Can you work these out from the model? Positions are in its coordinate system, mm. A direction names the side the tool comes from. Coordinates: 2 decimals unless noted, no trailing zeros. Loops run counter-clockwise (first coordinate to the right, second up) from the corner with the lowest first, then second, coordinate; pieces in that order, holes last.
```python
from build123d import *

# Parameters (mm, degrees)
BOSS_EXTRUDE1_DEPTH   = 17.78
BOSS_EXTRUDE1_2_DEPTH = 17.78
BOSS_EXTRUDE1_3_DEPTH = 17.78
BOSS_EXTRUDE1_4_DEPTH = 17.78
BOSS_EXTRUDE1_5_DEPTH = 17.78
BOSS_EXTRUDE1_6_DEPTH = 17.78
BOSS_EXTRUDE2_DEPTH   = 7.62


with BuildPart() as part:
    # Sketch1 → Boss-Extrude1 (new body)
    with BuildSketch(Plane.XY):
        with BuildLine():
            Line((-63.5, 0.762), (-38.022245391, 0.762))
            ThreePointArc((-38.022245391, 0.762), (-31.409051973, 4.854056156), (-32.119852619, 12.598345226))
            Line((-32.119852619, 12.598345226), (-38.427776706, 20.532214336))
            Line((-38.427776706, 20.532214336), (-27.33774172, 20.532214336))
            Line((-27.33774172, 20.532214336), (-27.33774172, 0.762))
            Line((-27.33774172, 0.762), (-17.932333685, 0.762))
            Line((-17.932333685, 0.762), (-17.932333685, 20.532214336))
            Line((-17.932333685, 20.532214336), (-7.881253338, 20.532214336))
            Line((-7.881253338, 20.532214336), (-7.881253338, 29.930214336))
            Line((-7.881253338, 29.930214336), (-42.276317647, 29.930214336))
            ThreePointArc((-42.276317647, 29.930214336), (-48.598760185, 24.736726392), (-47.348213221, 16.650829474))
            Line((-47.348213221, 16.650829474), (-42.18759625, 10.16))
            Line((-42.18759625, 10.16), (-63.5, 10.16))
            Line((-63.5, 10.16), (-63.5, 0.762))
        make_face()
    extrude(amount=BOSS_EXTRUDE1_DEPTH)



with BuildPart() as body_2:
    # Sketch1 → Boss-Extrude1 2 (new body)
    with BuildSketch(Plane.XY):
        Polygon((11.051079885, 6.067535635), (13.004416536, 0.762), (23.01912578, 0.762), (12.280277522, 29.930214336), (-2.050542709, 29.930214336), (-13.385046463, 0.762), (-3.302420584, 0.762), (-1.240737517, 6.067535635), align=None)
        Polygon((5.071020227, 22.310214336), (0.733304445, 11.147535635), (9.180778587, 11.147535635), align=None, mode=Mode.SUBTRACT)
    extrude(amount=BOSS_EXTRUDE1_2_DEPTH)


with BuildPart() as body_3:
    # Sketch1 → Boss-Extrude1 3 (new body)
    with BuildSketch(Plane.XY):
        with BuildLine():
            ThreePointArc((43.443733283, 11.869404165), (43.556066702, 11.637854646), (43.712774585, 11.43370613))
            Line((43.712774585, 11.43370613), (44.162226788, 10.95718914))
            ThreePointArc((44.162226788, 10.95718914), (45.003789062, 10.367797223), (46.009984972, 10.16))
            Line((46.009984972, 10.16), (73.255000443, 10.16))
            Line((73.255000443, 10.16), (73.255000443, 0.762))
            Line((73.255000443, 0.762), (46.72115082, 0.762))
            ThreePointArc((46.72115082, 0.762), (45.463753928, 0.920074253), (44.28460982, 1.384459427))
            Line((44.28460982, 1.384459427), (43.705112819, 1.7012189))
            ThreePointArc((43.705112819, 1.7012189), (40.598056426, 3.858045423), (38.01751427, 6.623276383))
            Line((38.01751427, 6.623276383), (33.528766448, 12.598345226))
            Line((33.528766448, 12.598345226), (33.528766448, 0.762))
            Line((33.528766448, 0.762), (23.991875044, 0.762))
            Line((23.991875044, 0.762), (23.991875044, 29.930214336))
            Line((23.991875044, 29.930214336), (33.521137043, 29.930214336))
            Line((33.521137043, 29.930214336), (43.884526544, 29.930214336))
            ThreePointArc((43.884526544, 29.930214336), (52.294019037, 20.754281762), (43.366111034, 12.081925607))
            Line((43.366111034, 12.081925607), (43.443733283, 11.869404165))
        make_face()
        with BuildLine():
            ThreePointArc((41.080111034, 18.914029667), (43.179680202, 21.013598834), (41.080111034, 23.113168002))
            Line((41.080111034, 23.113168002), (33.525986314, 23.113168314))
            Line((33.525986314, 23.113168314), (33.525986314, 18.914029667))
            Line((33.525986314, 18.914029667), (41.080111034, 18.914029667))
        make_face(mode=Mode.SUBTRACT)
    extrude(amount=BOSS_EXTRUDE1_3_DEPTH)


with BuildPart() as body_4:
    # Sketch1 → Boss-Extrude1 4 (new body)
    with BuildSketch(Plane.XY):
        with BuildLine():
            ThreePointArc((30.671195496, -18.911591325), (30.783528915, -19.143140844), (30.940236798, -19.347289359))
            Line((30.940236798, -19.347289359), (31.389689001, -19.82380635))
            ThreePointArc((31.389689001, -19.82380635), (32.231251275, -20.413198267), (33.237447184, -20.62099549))
            Line((33.237447184, -20.62099549), (54.549850935, -20.62099549))
            Line((54.549850935, -20.62099549), (49.389233963, -14.130166015))
            ThreePointArc((49.389233963, -14.130166015), (48.27077915, -5.719302433), (55.156904328, -0.762))
            Line((55.156904328, -0.762), (73.255000443, -0.762))
            Line((73.255000443, -0.762), (73.255000443, -10.248781153))
            Line((73.255000443, -10.248781153), (59.020836327, -10.248781153))
            Line((59.020836327, -10.248781153), (65.328760414, -18.182650263))
            ThreePointArc((65.328760414, -18.182650263), (66.03956106, -25.926939334), (59.426367642, -30.01899549))
            Line((59.426367642, -30.01899549), (33.948613033, -30.01899549))
            ThreePointArc((33.948613033, -30.01899549), (32.69121614, -29.860921236), (31.512072033, -29.396536062))
            Line((31.512072033, -29.396536062), (30.932575032, -29.079776589))
            ThreePointArc((30.932575032, -29.079776589), (27.825518639, -26.922950067), (25.244976483, -24.157719107))
            Line((25.244976483, -24.157719107), (20.756228661, -18.182650263))
            Line((20.756228661, -18.182650263), (20.756228661, -30.01899549))
            Line((20.756228661, -30.01899549), (11.219337256, -30.01899549))
            Line((11.219337256, -30.01899549), (11.219337256, -0.762))
            Line((11.219337256, -0.762), (31.111988756, -0.762))
            ThreePointArc((31.111988756, -0.762), (39.610601796, -10.010542083), (30.625924739, -18.787644819))
            Line((30.625924739, -18.787644819), (30.671195496, -18.911591325))
        make_face()
        with BuildLine():
            ThreePointArc((28.307573247, -12.053626898), (30.407142414, -9.954057774), (28.307573334, -7.854488563))
            Line((28.307573334, -7.854488563), (20.753448527, -7.85448825))
            Line((20.753448527, -7.85448825), (20.753448527, -12.053626898))
            Line((20.753448527, -12.053626898), (28.307573247, -12.053626898))
        make_face(mode=Mode.SUBTRACT)
    extrude(amount=BOSS_EXTRUDE1_4_DEPTH)


with BuildPart() as body_5:
    # Sketch1 → Boss-Extrude1 5 (new body)
    with BuildSketch(Plane.XY):
        Polygon((-1.719438494, -24.713459854), (0.233898158, -30.01899549), (10.246907832, -30.01899549), (-0.524626942, -0.762), (-14.788261104, -0.762), (-26.15726441, -30.01899549), (-16.072938963, -30.01899549), (-14.011255896, -24.713459854), align=None)
        Polygon((-7.701197721, -8.655916551), (-12.038913502, -19.818595252), (-3.591439361, -19.818595252), align=None, mode=Mode.SUBTRACT)
    extrude(amount=BOSS_EXTRUDE1_5_DEPTH)


with BuildPart() as body_6:
    # Sketch1 → Boss-Extrude1 6 (new body)
    with BuildSketch(Plane.XY):
        Polygon((-50.396276017, -10.825946893), (-53.629040398, -0.762), (-63.5, -0.762), (-54.102, -30.01899549), (-44.704, -30.01899549), (-41.933974753, -21.395605814), (-39.163949505, -30.01899549), (-29.765949505, -30.01899549), (-20.367949505, -0.762), (-30.238909107, -0.762), (-34.002210372, -12.477565879), (-37.765511637, -0.762), (-47.163511637, -0.762), align=None)
    extrude(amount=BOSS_EXTRUDE1_6_DEPTH)


with BuildPart() as part_1:
    add(part.part)

    add(body_2.part)  # Boss-Extrude2 merges body 2

    add(body_3.part)  # Boss-Extrude2 merges body 3

    add(body_4.part)  # Boss-Extrude2 merges body 4

    add(body_5.part)  # Boss-Extrude2 merges body 5

    add(body_6.part)  # Boss-Extrude2 merges body 6
    # Sketch2 → Boss-Extrude2 (add)
    with BuildSketch(Plane.XY):
        with BuildLine():
            Line((-55.151201275, -31.516967273), (-65.434483981, -0.083873468))
            Line((-65.434483981, -0.083873468), (-65.434483981, 12.305447779))
            Line((-65.434483981, 12.305447779), (-47.078741234, 12.305447779))
            Line((-47.078741234, 12.305447779), (-49.980640842, 15.906912471))
            ThreePointArc((-49.980640842, 15.906912471), (-51.234201523, 26.666707013), (-42.069273563, 32.441539344))
            Line((-42.069273563, 32.441539344), (46.103426171, 32.441539344))
            ThreePointArc((46.103426171, 32.441539344), (54.623601335, 23.874155401), (51.136703514, 12.305447779))
            Line((51.136703514, 12.305447779), (75.860238392, 12.305447779))
            Line((75.860238392, 12.305447779), (75.860238392, -11.870528257))
            Line((75.860238392, -11.870528257), (62.378876642, -11.870528257))
            Line((62.378876642, -11.870528257), (67.089261913, -17.64019673))
            ThreePointArc((67.089261913, -17.64019673), (68.184246101, -26.660573767), (60.504295946, -31.516967273))
            Line((60.504295946, -31.516967273), (-55.151201275, -31.516967273))
        make_face()
    extrude(amount=BOSS_EXTRUDE2_DEPTH)


solid = part_1.part
```
(1) If we mould it in two halves opening along X, with no side actions, what happens to faces 1 (the flat face through (-48.757, -5.724, 12.629)), 2 (the cylindrical face through (-48.555, 24.848, 12.629)), 3 (the flat face through (73.255, -5, 13)), 4 (the flat face through (5, 6.068, 13))? For each: released by +X, released by -X, zero draft, split by the parting line, or undercut.
Check values:
face 1: undercut
face 2: released by -X
face 3: released by +X
face 4: undercut
(2) I want a section at C-C on x = 6.5. Write out the boundary of the cut face in (y, z), then the cut area to 3 significant figures.
Check values:
outline: (-31.52, 0) - (32.44, 0) - (32.44, 7.62) - (29.93, 7.62) - (29.93, 17.78) - (18.43, 17.78) - (18.43, 7.62) - (11.15, 7.62) - (11.15, 17.78) - (6.07, 17.78) - (6.07, 7.62) - (-19.84, 7.62) - (-19.84, 17.78) - (-30.02, 17.78) - (-30.02, 7.62) - (-31.52, 7.62) - close
area: 759 mm2
(3) I want a section at B-B on z = 15.75. State how many separate pieces and enclosed holes the cut face has, then the cut area to 3 significant figures.
Check values:
separate pieces: 6
enclosed holes: 4
area: 5,260 mm2
(4) If I drill on probe 1 along X at (y, z) = (-24, 9.25); probe 2 along Y at (x, z) = (61, 15.75); probe 3 along X at (y, z) = (17, 15.5), over which ranges is the centre line in solid material (lowest first)?
Check values:
probe 1: x = -56.04 to -42.77, -41.1 to -27.83, -23.82 to 8.03, 11.22 to 20.76, 25.13 to 66.69
probe 2: y = -29.85 to -12.74, -10.25 to -0.76, 0.76 to 10.16
probe 3: x = -47.61 to -35.62, -27.34 to -17.93, -7.08 to 3.01, 7.03 to 17.04, 23.99 to 51.35
(5) I'm going to push flat-ended pins straight in: pin 1 (12 mm diameter, centred on x = -51, y = 9.5, fed in from -Z); pin 2 (5 mm diameter, centred on y = 15, z = 15, fed in from -X); pin 3 (10 mm diameter, centred on y = 26, z = 4, fed in from +X); pin 4 (8 mm diameter, centred on y = 22, z = 11.5, fed in from -X). Where does each tip first touch, or does it pass through?
Check values:
pin 1: stops at z = 0
pin 2: stops at x = -47.94
pin 3: stops at x = 54.98
pin 4: stops at x = -52.23
(6) I want a section at A-A on z = 2. Write out the boundary of the cut face in (x, y), then the cut area to 3 significant figures.
Check values:
outline: (-65.43, -0.08) - (-55.15, -31.52) - (60.5, -31.52) arc R8.5 ccw to (67.09, -17.64) - (62.38, -11.87) - (75.86, -11.87) - (75.86, 12.31) - (51.14, 12.31) arc R11.8 ccw to (46.1, 32.44) - (-42.07, 32.44) arc R10.16 ccw to (-49.98, 15.91) - (-47.08, 12.31) - (-65.43, 12.31) - close
area: 7,930 mm2
(7) I want a section at D-D on y = 14. Write out the boundary of the cut face in (x, z), then the cut area to 3 significant figures.
Check values:
outline: (-48.44, 0) - (52.66, 0) - (52.66, 7.62) - (48.9, 7.62) - (48.9, 17.78) - (23.99, 17.78) - (23.99, 7.62) - (18.15, 7.62) - (18.15, 17.78) - (8.13, 17.78) - (8.13, 7.62) - (1.84, 7.62) - (1.84, 17.78) - (-8.24, 17.78) - (-8.24, 7.62) - (-17.93, 7.62) - (-17.93, 17.78) - (-27.34, 17.78) - (-27.34, 7.62) - (-33.23, 7.62) - (-33.23, 17.78) - (-45.24, 17.78) - (-45.24, 7.62) - (-48.44, 7.62) - close
area: 1,450 mm2
(8) Which directions (+Z, -Z, +X, -X, +Y, -Y) give clear straight access to the entire face, cutting with the end or side of a thin tool? Please do faces 5 (the flat face through (21, -0.762, 13)), 6 (the flat face through (38, 21, 7.62)).
Check values:
face 5: +Z, +X, -X
face 6: +Z
